Design review of the part shown in the three views and the two pictorial views. Dimensions are in mm from the part's minimum x, y and z. A direction names the side the tool comes from. Coordinates: 2 decimals unless noted, no trailing zeros. Loops run counter-clockwise (first coordinate to the right, second up) from the corner with the lowest first, then second, coordinate; pieces in that order, holes last. Notation, with made-up numbers: (-24, 18) -> (-3, 18) arc R15 cw to (-3, 40) -> close; hole circle Ø7 at (12.5, 69.25). An arc over 180 degrees is marked (long way). Answer in a Markdown table with one row per item.
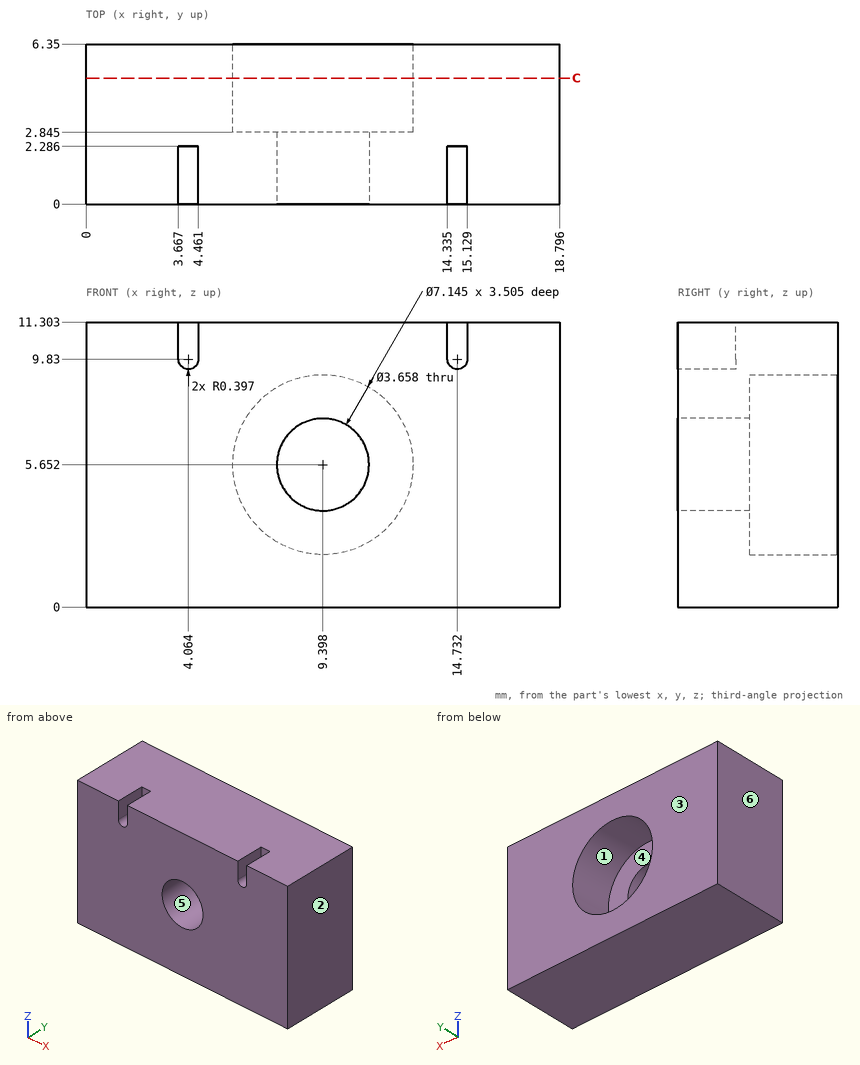
Item 1: Take a section at C-C, the plane y = 5. State the section outline as (x, z) points (1 decimal).
Worked answers:
| item | result |
|---|---|
| outline | (0, 0) -> (18.8, 0) -> (18.8, 11.3) -> (0, 11.3) -> close; hole circle Ø7.1 at (9.4, 5.7) |
Item 2: The part is to be moulded in two halves that separate along X. For the marked faces 3, 4, 5 and 6, say which applies: +X half, -X half, draft (parallel to the pull), parting line (faces both ways), or undercut.
Worked answers:
| item | result |
|---|---|
| face 3 | draft |
| face 4 | undercut |
| face 5 | undercut |
| face 6 | -X half |
Item 3: Insertion check: pin 1 (1.2 mm diameter, centred on y = 1, z = 10.5, fed in from -X); pin 2 (4.5 mm diameter, centred on x = 9.4, z = 5.65, fed in from +Y) (1 decimal). Each pin has a flat end and moves straight along its axis. Give the tip position at first contact, or say it passes through.
Worked answers:
| item | result |
|---|---|
| pin 1 | x = 0 |
| pin 2 | y = 2.8 |
Item 4: For L1, parallel to X at y = 0.5, z = 7.25 (1 decimal); L2, parallel to Z at x = 11.75, y = 4 (1 decimal); L3, parallel to Y at x = 10.25, z = 2.5 (1 decimal), list the stretches that pass through material, from the lowest coordinate up.
Worked answers:
| item | result |
|---|---|
| L1 | 0 to 8.5, 10.3 to 18.8 |
| L2 | 0 to 3, 8.3 to 11.3 |
| L3 | 0 to 2.8 |
Item 5: For the marked faces 1 and 2, list the 3-axis set-ups (+Z, -Z, +X, -X, +Y, -Y) from which the entire face can be reached by the end or side of a thin tool; tool diameter is ignored.
Worked answers:
| item | result |
|---|---|
| face 1 | +Y |
| face 2 | +Z, -Z, +X, +Y, -Y |
